Can you work these out from the model? Positions are in its coordinate system, mm. A direction names the side the tool comes from. Give positions to 0.01 mm unless a question says otherwise; leave off trailing zeros. Order: outer loops, then holes, each group sorted by start corner. A loop starts at its lowest first (then second) coordinate and runs counter-clockwise, first axis right, second up. Notation, with made-up numbers: (51, 51) - (82, 51) arc R19 cw to (82, 70) - close; hole circle Ø1 at (5, 27.5). An arc over 180 degrees is marked (long way). Write each question's results on one line, items separated by ' | '. Start each with the question number.
Autodesk Inventor part; units mm, degrees
ref_plane "作業平面1" through (0, 0, -38) normal (0, 1, 0) x (0, 0, 1)
ref_plane "YZ Plane" through (0, 0, 0) normal (1, 0, 0) x (0, 1, 0)
ref_plane "XZ Plane" through (0, 0, 0) normal (0, 1, 0) x (-1, 0, 0)
sketch "スケッチ1" plane through (0, 0, 0) normal (0, 1, 0) x (-1, 0, 0)
  line L0 (0, 0) -> (30, 0)
  line L1 (30, 0) -> (30, -135.2775)
  line L2 (30, -135.2775) -> (-78.1025, -135.2775)
  line L3 (-78.1025, -135.2775) -> (0, 0)
  dimension "d0" = 30
  dimension "d1" = 60
extrude "押し出し1" add sketch "スケッチ1" along normal blind 1.5
sketch "スケッチ2" plane through (0, 1.5, 0) normal (0, 1, 0) x (1, 0, 0)
  line L0 (-25, 8) -> (-25, 1.5)
  line L1 (-21.9199, 13.3349) -> (-25, 8)
  line L2 (-30, 18) -> (-21.9199, 13.3349)
  line L3 (-24.2265, 28) -> (-30, 18)
  line L4 (0, 28) -> (-24.2265, 28)
  line L5 (10.9697, 38) -> (0, 38)
  line L6 (13.5677, 36.5) -> (10.9697, 38)
  line L7 (11.0677, 32.1699) -> (13.5677, 36.5)
  line L8 (16.6969, 28.9199) -> (11.0677, 32.1699)
  line L9 (7.3612, 12.75) -> (16.6969, 28.9199)
  line L10 (0, 17) -> (7.3612, 12.75)
  line L11 (-12, 17) -> (0, 17)
  line L12 (-12, 8) -> (-12, 17)
  line L13 (-5, 8) -> (-12, 8)
  line L14 (-5, 1.5) -> (-5, 8)
  line L15 (-25, 1.5) -> (-5, 1.5)
  line L16 (78.1025, 135.2775) -> (-30, 135.2775)
  line L17 (-30, 135.2775) -> (-30, 0)
  line L18 (-30, 0) -> (0, 0)
  line L19 (0, 0) -> (78.1025, 135.2775)
  line L20 (-24.2265, 28) -> (-18.453, 38)
  line L21 (-18.453, 38) -> (5, 38)
  line L22 (13.5677, 36.5) -> (19.1969, 33.25)
  line L23 (0, 28) -> (0, 38)
  circle A0 centre (5, 34) radius 2.5
  circle A1 centre (5.5311, 19.5801) radius 1.35
  circle A2 centre (-16, 8) radius 1.35
  circle A3 centre (-22.5359, 22.9282) radius 1.35
  circle A4 centre (-6, 23) radius 1.35
  line L24 (-30, 1.5) -> (-25, 1.5)
  line L25 (-5, 1.5) -> (0.866, 1.5)
  point P0 (0, 36.5)
  point P1 (5, 36.5)
extrude "押し出し2" cut sketch "スケッチ2" against normal through all contours L15 L25 L19 L18 L17 L24 | L17 L16 L19 L22 L6 L5 L21 L20 L3
sketch "スケッチ3" plane through (0, 1.5, 0) normal (0, 1, 0) x (1, 0, 0)
  line L0 (-18.453, 38) -> (10.9697, 38)
  line L1 (5, 36.5) -> (-17, 36.5)
  line L2 (10.9697, 39) -> (-18.453, 39)
  line L3 (-18.453, 39) -> (-18.453, 35.5)
  line L4 (-18.453, 35.5) -> (10.9697, 35.5)
  line L5 (10.9697, 35.5) -> (10.9697, 39)
  line L6 (5, 36.5) -> (10.9697, 36.5)
  line L7 (-17, 36.5) -> (-18.453, 36.5)
  point P0 (0, 0)
  dimension "d6" = 1
  dimension "d7" = 1
extrude "押し出し3" add sketch "スケッチ3" against normal blind 3.5 contours L3 L2 L5 L0 | L7 L1 L6 L5 L4 L3
sketch "スケッチ4" plane through (0, 1.5, 0) normal (0, 1, 0) x (1, 0, 0)
  circle A0 centre (-16, 8) radius 1.6
  circle A1 centre (-22.5359, 22.9282) radius 1.6
  circle A2 centre (5.5311, 19.5801) radius 1.6
  circle A3 centre (5, 34) radius 1.6
  line L0 (0, 36.5) -> (0, 17)
  line L1 (-12, 8) -> (-12, 28)
  line L2 (-18.453, 38) -> (-30, 18)
  line L3 (-30, 18) -> (-21.9199, 13.3349)
  line L4 (0, 17) -> (7.3612, 12.75)
  line L5 (0.866, 1.5) -> (19.1969, 33.25)
  line L6 (10.9697, 39) -> (-18.453, 39)
  circle A4 centre (5, 34) radius 2.5
  point P0 (0, 0)
  point P1 (16.6969, 28.9199)
  dimension "d10" = 3.2
  dimension "d11" = 3.2
  dimension "d12" = 3.2
  dimension "d13" = 3.2
  dimension "d14" = 4
  dimension "d15" = 4
  dimension "d16" = 8
  dimension "d17" = 5
  dimension "d18" = 5
extrude "押し出し4" cut sketch "スケッチ4" against normal through all contours A0 | A1 | A2 | A3
sketch "スケッチ5" plane through (0, -2, 0) normal (0, -1, 0) x (1, 0, 0)
  line L0 (10.9697, -39) -> (3.9697, -39)
  line L1 (3.9697, -39) -> (3.9697, -35.5)
  line L2 (3.9697, -35.5) -> (10.9697, -35.5)
  line L3 (10.9697, -35.5) -> (10.9697, -39)
  line L4 (10.9697, -35.5) -> (5.5568, -35.5)
  point P0 (0, 0)
  dimension "d23" = 7
extrude "押し出し5" cut sketch "スケッチ5" against normal up to surface (2 mm away)
sketch "スケッチ6" plane through (0, -2, 0) normal (0, -1, 0) x (1, 0, 0)
  line L0 (-18.453, -36.5) -> (3.9697, -36.5)
  line L1 (3.9697, -36.5) -> (3.9697, -35.5)
  line L2 (3.9697, -35.5) -> (-18.453, -35.5)
  line L3 (-1.0303, -36.5) -> (-1.0303, -35.5)
  point P0 (0, 0)
  dimension "d26" = 5
ref_plane "作業平面1" through (0, 0, -38) normal (0, 1, 0) x (0, 0, 1)
extrude "押し出し6" cut sketch "スケッチ6" against normal up to surface (2 mm away)
properties part number "rail_cover_upper"
Q1. Which directions (+Z, -Z, +X, -X, +Y, -Y) give clear straight access to the entire face, cutting with the end or side of a thin tool? Please do faces 1 (the flat face through (-18.453, -0.2, -38.5)), 2 (the flat face through (10.97, 0.8, -38.5)), 3 (the flat face through (3.97, -1, -38.5)), 4 (the flat face through (-7, -1, -38)), 5 (the flat face through (-18.453, -1, -36)).
Q2. If we section it at A-A (x = -16): Please give me the cut outline in (y, z).
Q3. If we section it at B-B (x = -6): Please give me the cut outline in (y, z), plus the area to 4 significant figures.
Q4. If I drill on probe 1 along Z at (x, y) = (5, 0.5); probe 2 along Z at (x, y) = (-18, -1.35); probe 3 along Z at (x, y) = (-16, 1.1), over which ranges is the centre line in solid material (lowest first)? Write a range as from..to.
Q5. Will these pins go through, and if not, where does the flat tip stop? P1, Ø1.6, axis at x = -12, y = -1, coming from the +Z side; P2, Ø1.5, axis at y = -0.5, z = -26.5, coming from the -X side; P3, Ø1.1, axis at y = -1.5, z = -38.5, coming from the +X side.
Q6. Thinking about a two-plate mould opening in Z: for faces 6 (the flat face through (-10, -1, -36.5)), 7 (the flat face through (-1.03, -1, -36)), 8 (the flat face through (-4, 0, -39)), which applies, released by +Z, released by -Z, zero draft, split by the parting line, or undercut?
Q7. If we section it at D-D (y = 0.8): Please give me the cut outline in (x, z).
Q8. If we section it at C-C (z = -8): Please give me the cut outline in (x, y).
Findings below:
1) face 1: -Z, -X, +Y, -Y | face 2: -Z, +X, +Y, -Y | face 3: +Z, -Z, +X, -Y | face 4: +X, -X, -Y | face 5: +Z, -Z, -X, -Y
2) outline: (-2, -39) - (1.5, -39) - (1.5, -9.6) - (0, -9.6) - (0, -35.5) - (-2, -35.5) - (-2, -36.5) - (0, -36.5) - (0, -38) - (-2, -38) - close; (0, -6.4) - (1.5, -6.4) - (1.5, -1.5) - (0, -1.5) - close
3) outline: (-2, -39) - (1.5, -39) - (1.5, -1.5) - (0, -1.5) - (0, -35.5) - (-2, -35.5) - (-2, -36.5) - (0, -36.5) - (0, -38) - (-2, -38) - close | area: 60.25 mm2
4) probe 1: z = -39..-35.6, -32.4..-21.09, -18.07..-8.66 | probe 2: z = -39..-38, -36.5..-35.5 | probe 3: z = -39..-9.6, -6.4..-1.5
5) P1: stops at z = -35.5 | P2: stops at x = -25.42 | P3: stops at x = 3.97
6) face 6: undercut | face 7: zero draft | face 8: released by -Z
7) outline: (-30, -18) - (-18.45, -38) - (-18.45, -39) - (10.97, -39) - (10.97, -38) - (13.57, -36.5) - (19.2, -33.25) - (0.87, -1.5) - (-30, -1.5) - close; hole circle Ø3.2 at (-22.54, -22.93); hole circle Ø3.2 at (-16, -8); hole circle Ø3.2 at (5, -34); hole circle Ø3.2 at (5.53, -19.58)
8) outline: (-30, 0) - (-17.6, 0) - (-17.6, 1.5) - (-30, 1.5) - close; (-14.4, 0) - (4.62, 0) - (4.62, 1.5) - (-14.4, 1.5) - close
